from build123d import *

# Parameters (mm, degrees)
SKETCH1_W           = 131
SKETCH1_H           = 66
BOSS_EXTRUDE1_DEPTH = 5
FILLET1_R           = 3
SKETCH2_R           = 2.25
CUT_EXTRUDE1_DEPTH  = 74.513604183
SKETCH3_W           = 100
SKETCH3_H           = 50
CUT_EXTRUDE2_DEPTH  = 3.2
SKETCH4_W           = 88
SKETCH4_H           = 38
CUT_EXTRUDE3_DEPTH  = 74.413145962


with BuildPart() as part:
    # Sketch1 → Boss-Extrude1 (new body)
    with BuildSketch(Plane(origin=(0, 0, 0), x_dir=(1, 0, 0), z_dir=(0, 1, 0))):
        Rectangle(SKETCH1_W, SKETCH1_H)
    extrude(amount=BOSS_EXTRUDE1_DEPTH)

    # Fillet1
    fillet1_edges = [part.edges().sort_by_distance(p)[0] for p in [
        (65.5, 2.5, 33),
        (-65.5, 2.5, 33),
        (-65.5, 2.5, -33),
        (65.5, 2.5, -33),
    ]]
    fillet(fillet1_edges, radius=FILLET1_R)

    # Sketch2 → Cut-Extrude1 (cut, through all)
    with BuildSketch(Plane(origin=(0, 5, 0), x_dir=(1, 0, 0), z_dir=(0, 1, 0))):
        with Locations(Location((-61.5, 29, 0), (0, 0, 270))):
            Circle(SKETCH2_R)
        with Locations(Location((61.5, 29, 0), (0, 0, 270))):
            Circle(SKETCH2_R)
        with Locations(Location((61.5, -29, 0), (0, 0, 270))):
            Circle(SKETCH2_R)
        with Locations(Location((-61.5, -29, 0), (0, 0, 270))):
            Circle(SKETCH2_R)
        with Locations(Location((0, 29, 0), (0, 0, 270))):
            Circle(SKETCH2_R)
        with Locations(Location((0, -29, 0), (0, 0, 270))):
            Circle(SKETCH2_R)
    extrude(amount=-CUT_EXTRUDE1_DEPTH, mode=Mode.SUBTRACT)

    # Sketch3 → Cut-Extrude2 (cut)
    with BuildSketch(Plane(origin=(0, 5, 0), x_dir=(1, 0, 0), z_dir=(0, 1, 0))):
        Rectangle(SKETCH3_W, SKETCH3_H)
    extrude(amount=-CUT_EXTRUDE2_DEPTH, mode=Mode.SUBTRACT)

    # Sketch4 → Cut-Extrude3 (cut, through all)
    with BuildSketch(Plane(origin=(0, 1.8, 0), x_dir=(1, 0, 0), z_dir=(0, 1, 0))):
        Rectangle(SKETCH4_W, SKETCH4_H)
    extrude(amount=-CUT_EXTRUDE3_DEPTH, mode=Mode.SUBTRACT)


solid = part.part
Design review of the part built by this model. Coordinates are the model's own, in mm. A direction names the side the tool comes from. Round coordinates to 2 decimals unless told otherwise and drop trailing zeros. Write each loop counter-clockwise with the first axis right and the second up, starting at its lowest first coordinate (ties: lowest second). Pieces come first, ordered by that corner, then holes. Notation, with made-up numbers: (49.5, 25) -> (98.5, 25) arc R32 ccw to (98.5, 55) -> close; hole circle Ø2 at (28.5, 38.5). An arc over 180 degrees is marked (long way). One line per question, with ' | ' between items.
(1) Take a section at A-A, the plane x = -17. State the section outline as (y, z) points.
Result sheet:
outline: (0, -33) -> (5, -33) -> (5, -25) -> (1.8, -25) -> (1.8, -19) -> (0, -19) -> close; (0, 19) -> (1.8, 19) -> (1.8, 25) -> (5, 25) -> (5, 33) -> (0, 33) -> close
(2) Insertion check: P1, Ø2.5, axis at x = 61.5, z = -29, coming from the +Y side; P2, Ø6, axis at x = -61.5, z = -29, coming from the +Y side. Each pin has a flat end and moves straight along its axis. Give the tip position at first contact, or say it passes through.
Result sheet:
P1: through | P2: y = 5
(3) Take a section at C-C, the plane y = 4.15. State the section outline as (x, z) points, and give its area (3 significant figures).
Result sheet:
outline: (-65.5, -30) arc R3 ccw to (-62.5, -33) -> (62.5, -33) arc R3 ccw to (65.5, -30) -> (65.5, 30) arc R3 ccw to (62.5, 33) -> (-62.5, 33) arc R3 ccw to (-65.5, 30) -> close; hole circle Ø4.5 at (-61.5, -29); hole circle Ø4.5 at (-61.5, 29); hole (-50, -25) -> (50, -25) -> (50, 25) -> (-50, 25) -> close; hole circle Ø4.5 at (0, -29); hole circle Ø4.5 at (0, 29); hole circle Ø4.5 at (61.5, -29); hole circle Ø4.5 at (61.5, 29) | area: 3,540 mm2
(4) Machinability: for faces 1 (the flat face through (50, 3, 0)), 2 (the cylindrical face through (59.504, 2.535, 30.038)), which of the approach directions +Z, -Z, +X, -X, +Y, -Y give a long, thin tool a straight path to every point of the face, cutting with its end or side? Answer none if there is none.
Result sheet:
face 1: +Y | face 2: +Y, -Y
(5) Take a section at D-D, the plane x = 0. State the section outline as (y, z) points, and give its area (3 significant figures).
Result sheet:
outline: (0, -33) -> (5, -33) -> (5, -31.25) -> (0, -31.25) -> close; (0, -26.75) -> (5, -26.75) -> (5, -25) -> (1.8, -25) -> (1.8, -19) -> (0, -19) -> close; (0, 19) -> (1.8, 19) -> (1.8, 25) -> (5, 25) -> (5, 26.75) -> (0, 26.75) -> close; (0, 31.25) -> (5, 31.25) -> (5, 33) -> (0, 33) -> close | area: 56.6 mm2
(6) Wall thickness on line 1 (X direction, y = 2.8, z = 29); line 2 (X direction, y = 2.4, z = 6); line 3 (Z direction, x = 5.5, y = 2.75): over which ranges is each line inside the solid? List them lowest first. Write a range as [from, to].
Result sheet:
line 1: [-65.5, -63.75], [-59.25, -2.25], [2.25, 59.25], [63.75, 65.5] | line 2: [-65.5, -50], [50, 65.5] | line 3: [-33, -25], [25, 33]
(7) Take a section at B-B, the plane z = 8.5. State the section outline as (x, y) points.
Result sheet:
outline: (-65.5, 0) -> (-44, 0) -> (-44, 1.8) -> (-50, 1.8) -> (-50, 5) -> (-65.5, 5) -> close; (44, 0) -> (65.5, 0) -> (65.5, 5) -> (50, 5) -> (50, 1.8) -> (44, 1.8) -> close
